Verification items for the finished model (mm, model axes). Give positions to 0.01 mm unless a question says otherwise; leave off trailing zeros. Write each loop counter-clockwise with the first axis right and the second up, starting at its lowest first coordinate (ties: lowest second). Pieces come first, ordered by that corner, then holes.
from build123d import *

# Parameters (mm, degrees)
SKETCH1_R           = 1.75
BOSS_EXTRUDE1_DEPTH = 4
FILLET1_R           = 4


with BuildPart() as part:
    # Sketch1 → Boss-Extrude1 (new body)
    with BuildSketch(Plane(origin=(0, 0, 0), x_dir=(0, 0, -1), z_dir=(1, 0, 0))):
        Polygon((35, 25), (95, 25), (95, -25), (-95, -25), (-95, 25), (-35, 25), (-35, 165), (35, 165), align=None)
        with Locations((0, 145)):
            Circle(SKETCH1_R, mode=Mode.SUBTRACT)
        with Locations((0, 125)):
            Circle(SKETCH1_R, mode=Mode.SUBTRACT)
        with Locations((0, 105)):
            Circle(SKETCH1_R, mode=Mode.SUBTRACT)
    extrude(amount=BOSS_EXTRUDE1_DEPTH)

    # Fillet1
    fillet1_edges = [part.edges().sort_by_distance(p)[0] for p in [
        (2, 25, 35),
        (2, 165, 35),
        (2, 165, -35),
        (2, 25, -35),
    ]]
    fillet(fillet1_edges, radius=FILLET1_R)


solid = part.part
Item 1: Depth check by flat-ended pin: pin 1 (1.5 mm diameter, centred on x = 3, y = 94, fed in from -Z); pin 2 (2 mm diameter, centred on x = 2, z = 53.5, fed in from +Y). Enter the tip coordinate at first touch or a pass-through.
Answer key:
pin 1: stops at z = -35
pin 2: stops at y = 25
Item 2: Sectioned sample at A-A on x = 2.5. Record the cut outline in (y, z), then the cut area to 3 significant figures.
Answer key:
outline: (-25, -95) - (25, -95) - (25, -39) arc R4 cw to (29, -35) - (161, -35) arc R4 ccw to (165, -31) - (165, 31) arc R4 ccw to (161, 35) - (29, 35) arc R4 cw to (25, 39) - (25, 95) - (-25, 95) - close; hole circle Ø3.5 at (105, 0); hole circle Ø3.5 at (125, 0); hole circle Ø3.5 at (145, 0)
area: 19,300 mm2
Item 3: Sectioned sample at C-C on y = 98. Record the cut outline in (x, z).
Answer key:
outline: (0, -35) - (4, -35) - (4, 35) - (0, 35) - close
Item 4: Scan lines: line 1 along Y through (x, z) = (2.4, 0); line 2 along Z through (x, y) = (1.35, 105); line 3 along Z through (x, y) = (2.65, 38). Record each from-to range of solid material in increasing order.
Answer key:
line 1: y = -25 to 103.25, 106.75 to 123.25, 126.75 to 143.25, 146.75 to 165
line 2: z = -35 to -1.75, 1.75 to 35
line 3: z = -35 to 35
Item 5: Sectioned sample at B-B on z = -83. Record the cut outline in (x, y).
Answer key:
outline: (0, -25) - (4, -25) - (4, 25) - (0, 25) - close
